Autodesk Inventor part; units mm, degrees
ref_plane "Work Plane1" through (32.4111, 0, 0) normal (0, 0, -1) x (-1, 0, 0)
ref_plane "YZ Plane" through (0, 0, 0) normal (1, 0, 0) x (0, 1, 0)
ref_plane "XZ Plane" through (0, 0, 0) normal (0, 1, 0) x (-1, 0, 0)
sketch "Sketch1" plane through (0, 0, 0) normal (0, 0, 1) x (1, 0, 0)
  line L0 (-2.3453, 0) -> (12.0575, 0)
  line L1 (4.329, 7.5) -> (2.799, 10.15)
  line L2 (4.329, 7.5) -> (10, 7.5) construction
  line L3 (10, 7.5) -> (10, 0) construction
  arc A0 (2.799, 10.15) -> (0, 9.4) centre (1.5, 9.4) ccw
  line L4 (4.329, 7.5) -> (4.329, 0)
  line L5 (0, -2.2448) -> (0, 13.4687)
  point P0 (0, 0)
  dimension "d2" = 15
  dimension "d4" = 21.8
  dimension "d5" = 1.5
  dimension "d15" = 10
  dimension "d16" = 30
revolve "Ring" add sketch "Sketch1" angle 360 about axis through (-10, 0, 0) along (1, 0, 0)
sketch "Sketch2" plane through (0, 0, 0) normal (-1, 0, 0) x (0, 0, 1)
  circle A0 centre (0, 0) radius 4.9
  line L0 (-7.5, -4.3301) -> (-7.5, 4.3301)
  line L1 (-7.5, 4.3301) -> (0, 8.6603)
  line L2 (0, 8.6603) -> (7.5, 4.3301)
  line L3 (7.5, 4.3301) -> (7.5, -4.3301)
  line L4 (7.5, -4.3301) -> (0, -8.6603)
  line L5 (0, -8.6603) -> (-7.5, -4.3301)
  circle A1 centre (0, 0) radius 9.4
  dimension "d6" = 17.3205
extrude "Body" add sketch "Sketch2" against normal blind 10 contours A0 | L0 L1 L2 L3 L4 L5
sketch "Sketch3" plane through (0, 0, 0) normal (0, 0, 1) x (1, 0, 0)
  line L0 (3.6591, 8.6603) -> (10, 8.6603)
  line L1 (10, 4.3301) -> (10, 8.6603)
  line L2 (0, -9.4) -> (0, 9.4)
  line L3 (-2, 0) -> (12, 0)
  line L4 (9.3301, 8.6603) -> (10, 7.5)
  dimension "d10" = 30
  dimension "d11" = 15
revolve "Chamfer1" cut sketch "Sketch3" angle 360 about axis through (-10, 0, 0) along (1, 0, 0)
sketch "Sketch4" plane through (0, 0, 0) normal (-1, 0, 0) x (0, 0, 1)
  circle A0 centre (0, 0) radius 9.4
hole "Thread" at (0, 0, 0) direction (1, 0, 0) diameter 8.376 end through all
chamfer "Chamfer2" distance 0.8119 angle 30 1 edges at (0, 0, -4.188) measured on face at (0, 7.5614, -0.9181)
ref_plane "Work Plane1" through (32.4111, 0, 0) normal (0, 0, -1) x (-1, 0, 0)
chamfer "Chamfer3" distance 0.8119 angle 45 1 edges at (10, 0, -4.188)
equation "\"d2\" = SW"
equation "\"d4\" = LADI"
equation "\"d5\" = PHH"
equation "\"d15\" = KOH"
equation "\"d16\" = KEWI"
equation "\"d6\" = 1.1547 * SW"
equation "\"d7\" = KOH"
equation "\"d10\" = ANG1"
equation "\"d11\" = SW0"
equation "\"d12\" = -0.5 * GD1 + 0.5 * NND"
equation "\"d46\" = -0.5 * GD1 + 0.5 * NND"
equation "\"d51\" = -0.5 * GD1 + 0.5 * NND"
equation "\"ANG1\" = 30deg"
equation "\"KEWI\" = 30deg"
equation "\"LADI\" = 21.8"
equation "\"SW\" = 15"
equation "\"PHH\" = RR"
equation "\"KOH\" = 10"
equation "\"SW0\" = SW"
equation "\"d1\" = LADI"
equation "\"d3\" = PHH"
equation "\"GUL\" = 0.541266 * PTC"
equation "\"RR\" = 1.5"
equation "\"TOA\" = 30deg"
equation "\"PTC\" = 1.5"
equation "\"RR1\" = 0.6"
equation "\"GAL\" = 0.541266 * PTC"
equation "\"E0\" = 1.155 * SW"
properties part number "ANSI B18.2.4.4M - M10 x 1,5" material "Steel, Mild"
Input: part model. Units: mm. Frame: model coordinates. A direction names the side the tool comes from. Give positions to 0.01 mm unless a question says otherwise; leave off trailing zeros. Write each loop counter-clockwise with the first axis right and the second up, starting at its lowest first coordinate (ties: lowest second). Pieces come first, ordered by that corner, then holes.
Q1. Material intervals for probe 1 along Z at (x, y) = (5.5, 0); probe 2 along Y at (x, z) = (6.75, 3.5); probe 3 along Z at (x, y) = (3.5, 0), sorted ascending.
Q2. Pull-direction query (Y, two-part tool) for faces 4 (the face through (7, 0, 7.5)), 5 (the face through (4.889, -2.83, -3.087)), 6 (the face through (4.063, 7.593, -2.391)), 7 (the face through (9.84, -7.78, -0.02)); classes: pulls with the +Y half, pulls with the -Y half, needs draft (parallel to the pull), parting line crosses it, or undercut.
Q3. Section A-A, the plane x = 4. Output: boundary loops of the cut face in (y, z).
Q4. Set-up query: faces 1 (the face through (6.785, 6.526, 3.698)), 2 (the face through (6.785, 6.465, -3.803)), 3 (the face through (6.785, -6.526, -3.698)). Return all of +Z, -Z, +X, -X, +Y, -Y with unobstructed straight access to the full face (end or side cutting, diameter ignored); none if empty.
Q5. First-contact query: P1, Ø2, axis at x = 1, z = -3.5, coming from the +Y side; P2, Ø2, axis at y = 8.5, z = -7.5, coming from the -X side; P3, Ø1, axis at x = 7.5, z = -5, coming from the -Y side; P4, Ø3, axis at y = -6, z = -7, coming from the -X side. Flat tips, straight axial feed; report the tip coordinate or a pass-through.
Filled in:
1. probe 1: z = -7.5 to -4.19, 4.19 to 7.5
1. probe 2: y = -6.64 to -2.3, 2.3 to 6.64
1. probe 3: z = -8.94 to -4.19, 4.19 to 8.94
2. face 4: needs draft
2. face 5: undercut
2. face 6: parting line crosses it
2. face 7: pulls with the -Y half
3. outline: (-8.66, 0) - (-7.98, -1.17) arc R8.07 ccw to (-5.01, -6.33) - (-4.33, -7.5) - (-2.98, -7.5) arc R8.07 ccw to (2.98, -7.5) - (4.33, -7.5) - (5.01, -6.33) arc R8.07 ccw to (7.98, -1.17) - (8.66, 0) - (7.98, 1.17) arc R8.07 ccw to (5.01, 6.33) - (4.33, 7.5) - (2.98, 7.5) arc R8.07 ccw to (-2.98, 7.5) - (-4.33, 7.5) - (-5.01, 6.33) arc R8.07 ccw to (-7.98, 1.17) - close; hole circle Ø8.38 at (0, 0)
4. face 1: +Z, +X, +Y
4. face 2: -Z, +X, +Y
4. face 3: -Z, +X, -Y
5. P1: stops at y = 10.59
5. P2: stops at x = 0.33
5. P3: stops at y = -6.06
5. P4: stops at x = 0
